The model under review builds one solid part; all positions refer to its coordinate system, in mm. A direction names the side the tool comes from. Round coordinates to 2 decimals unless told otherwise and drop trailing zeros. Order: outer loops, then holes, each group sorted by start corner. A loop starts at its lowest first (then second) coordinate and runs counter-clockwise, first axis right, second up. Notation, with made-up numbers: (-25, -13.75) -> (21, -13.75) arc R33 ccw to (21, 21.25) -> close; hole circle Ø1 at (51, 57). An arc over 180 degrees is marked (long way). Use a Markdown table: item, result. Add a question column.
```python
from build123d import *

# Parameters (mm, degrees)
PAD_DEPTH       = 28
SKETCH001_R     = 19
POCKET_DEPTH    = 5
POCKET001_DEPTH = 26
SKETCH003_W     = 30
SKETCH003_H     = 6
POCKET002_DEPTH = 10
SKETCH004_W     = 2.8
SKETCH004_H     = 40
PAD001_DEPTH    = 5.8
SKETCH005_W     = 2.722469
SKETCH005_H     = 3
SKETCH005_W_2   = 2.715425
PAD002_DEPTH    = 12
SKETCH006_R     = 1.6
POCKET003_DEPTH = 5
SKETCH007_W     = 1
SKETCH007_H     = 4
POCKET004_DEPTH = 6
PAD003_DEPTH    = 10
SKETCH009_W     = 14.845783
SKETCH009_H     = 0.4
POCKET005_DEPTH = 0.4


with BuildPart() as part:
    # Sketch → Pad (new body)
    with BuildSketch(Plane(origin=(0, 0, 0), x_dir=(1, 0, 0), z_dir=(0, 0, -1))):
        Polygon((-52.483848, 11.054775), (-10.483848, 11.054775), (-10.483848, 16.054775), (-24.483848, 32.054775), (-38.483848, 32.054775), (-52.483848, 16.054775), align=None)
    extrude(amount=PAD_DEPTH)

    # Sketch001 → Pocket (cut)
    with BuildSketch(Plane(origin=(0, -11.054775, 0), x_dir=(1, 0, 0), z_dir=(0, 1, 0))):
        with Locations((-31.483848, 21)):
            Circle(SKETCH001_R)
    extrude(amount=-POCKET_DEPTH, mode=Mode.SUBTRACT)

    # Sketch002 → Pocket001 (cut)
    with BuildSketch(Plane(origin=(0, 0, -28), x_dir=(1, 0, 0), z_dir=(0, 0, -1))):
        Polygon((-49.14737, 16.054775), (-36.483848, 32.054775), (-26.483848, 32.054775), (-13.820326, 16.054775), align=None)
    extrude(amount=-POCKET001_DEPTH, mode=Mode.SUBTRACT)

    # Sketch003 → Pocket002 (cut)
    with BuildSketch(Plane(origin=(0, 0, -28), x_dir=(1, 0, 0), z_dir=(0, 0, -1))):
        with Locations((-31.483848, 29.054775)):
            Rectangle(SKETCH003_W, SKETCH003_H)
    extrude(amount=-POCKET002_DEPTH, mode=Mode.SUBTRACT)

    # Sketch004 → Pad001 (new body)
    with BuildSketch(Plane(origin=(0, 0, -28), x_dir=(1, 0, 0), z_dir=(0, 0, -1))):
        with Locations((-46.98737, 40.454775)):
            Rectangle(SKETCH004_W, SKETCH004_H)
        with Locations((-15.98737, 40.454775)):
            Rectangle(SKETCH004_W, SKETCH004_H)
    extrude(amount=-PAD001_DEPTH)

    # Sketch005 → Pad002 (new body)
    with BuildSketch(Plane(origin=(0, 0, -28), x_dir=(1, 0, 0), z_dir=(0, 0, -1))):
        with Locations((-47.026135, 21.954775)):
            Rectangle(SKETCH005_W, SKETCH005_H)
        with Locations((-15.945082, 21.954775)):
            Rectangle(SKETCH005_W_2, SKETCH005_H)
    extrude(amount=-PAD002_DEPTH)

    # Sketch006 → Pocket003 (cut)
    with BuildSketch(Plane(origin=(0, -11.054775, 0), x_dir=(1, 0, 0), z_dir=(0, 1, 0))):
        with Locations((-47.483848, 4)):
            Circle(SKETCH006_R)
        with Locations((-15.483848, 4)):
            Circle(SKETCH006_R)
    extrude(amount=-POCKET003_DEPTH, mode=Mode.SUBTRACT)

    # Sketch007 → Pocket004 (cut)
    with BuildSketch(Plane(origin=(0, 0, -28), x_dir=(1, 0, 0), z_dir=(0, 0, -1))):
        with Locations((-46.98737, 55.054775)):
            Rectangle(SKETCH007_W, SKETCH007_H)
        with Locations((-15.98737, 55.054775)):
            Rectangle(SKETCH007_W, SKETCH007_H)
    extrude(amount=-POCKET004_DEPTH, mode=Mode.SUBTRACT)

    # Sketch008 → Pad003 (new body)
    with BuildSketch(Plane(origin=(0, 0, -18), x_dir=(1, 0, 0), z_dir=(0, 0, -1))):
        Polygon((-32.222141, 44.054382), (-31.422141, 44.054382), (-31.422141, 32.054775), (-24.483848, 32.054775), (-24.483848, 31.254775), (-38.483848, 31.254775), (-38.483848, 32.054775), (-32.222141, 32.054775), align=None)
    extrude(amount=PAD003_DEPTH)

    # Sketch009 → Pocket005 (cut)
    with BuildSketch(Plane(origin=(0, -31.254775, 0), x_dir=(1, 0, 0), z_dir=(0, 1, 0))):
        with Locations((-31.447088, 18.2)):
            Rectangle(SKETCH009_W, SKETCH009_H)
    extrude(amount=-POCKET005_DEPTH, mode=Mode.SUBTRACT)


solid = part.part
```
Q1. Add section A-A, the plane z = -21. Give the number of separate pieces and of enclosed holes in the cut face, then the cut area to 3 significant figures.
Q2. Add section D-D, the plane z = -4. Give the boundary of the cut face in (x, y), then the cut area to 3 significant figures.
Q3. For pin 1 (4.5 mm diameter, centred on y = -49.5, z = -24, fed in from +X); pin 2 (6 mm diameter, centred on x = -43.5, z = -7, fed in from -Y); pin 3 (2 mm diameter, centred on x = -21, z = -22.5, fed in from -Y), all flat-tipped, find the tip position at first contact; note any pin that passes through.
Q4. Draft analysis for pull direction X (two halves, no side actions). For faces 5 (the face through (-32.222, -38, -23)), 6 (the face through (-32, -35, -28)), 7 (the face through (-33, -32.055, -20)), 8 (the face through (-10.484, -14, -14)), state which applies: released by +X, released by -X, zero draft, split by the parting line, or undercut.
Q5. Add section C-C, the plane y = -33. Give the boundary of the cut face in (x, z), then the cut area to 3 significant figures.
Q6. To check wall thickness, follow line 1 along X through (y, z) = (-13.35, -21); line 2 along X through (y, z) = (-14.1, -4); line 3 along Z through (x, y) = (-34.5, -29). State the ranges of each line that lie inside material, in increasing order.
Q7. For faces 1 (the face through (-14.587, -22, -22)), 2 (the face through (-15.487, -55, -25)), 3 (the face through (-48.387, -22, -19)), 4 (the face through (-32.002, -13.52, -2.007)), list the 3-axis set-ups (+Z, -Z, +X, -X, +Y, -Y) from which the entire face can be reached by the end or side of a thin tool; tool diameter is ignored.
Q8. Add section B-B, the plane y = -55.5. Give the boundary of the cut face in (x, z), then the cut area to 3 significant figures.
Return value:
| question | item | result |
|---|---|---|
| 1 | separate pieces | 3 |
| 1 | enclosed holes | 0 |
| 1 | area | 106 mm² |
| 2 | outline | (-52.48, -16.05) -> (-38.48, -32.05) -> (-36.48, -32.05) -> (-49.15, -16.05) -> (-49.08, -16.05) -> (-49.08, -11.05) -> (-52.48, -11.05) -> close; (-45.88, -16.05) -> (-39.97, -16.05) -> (-39.97, -11.05) -> (-45.88, -11.05) -> close; (-26.48, -32.05) -> (-24.48, -32.05) -> (-10.48, -16.05) -> (-10.48, -11.05) -> (-13.88, -11.05) -> (-13.88, -16.05) -> (-13.82, -16.05) -> close; (-23, -16.05) -> (-17.08, -16.05) -> (-17.08, -11.05) -> (-23, -11.05) -> close |
| 2 | area | 179 mm² |
| 3 | pin 1 | x = -14.59 |
| 3 | pin 2 | y = -29.75 |
| 3 | pin 3 | y = -26.05 |
| 4 | face 5 | undercut |
| 4 | face 6 | zero draft |
| 4 | face 7 | undercut |
| 4 | face 8 | released by +X |
| 5 | outline | (-48.39, -28) -> (-45.59, -28) -> (-45.59, -22.2) -> (-48.39, -22.2) -> close; (-32.22, -28) -> (-31.42, -28) -> (-31.42, -18) -> (-32.22, -18) -> close; (-17.39, -28) -> (-14.59, -28) -> (-14.59, -22.2) -> (-17.39, -22.2) -> close |
| 5 | area | 40.5 mm² |
| 6 | line 1 | -52.48 to -50.48, -12.48 to -10.48 |
| 6 | line 2 | -52.48 to -49.08, -45.88 to -39.97, -23 to -17.08, -13.88 to -10.48 |
| 6 | line 3 | -2 to 0 |
| 7 | face 1 | +Z, -Z, +X, -Y |
| 7 | face 2 | +Z, -Z |
| 7 | face 3 | +Z, -Z, -X, -Y |
| 7 | face 4 | +Y |
| 8 | outline | (-48.39, -28) -> (-47.49, -28) -> (-47.49, -22.2) -> (-48.39, -22.2) -> close; (-46.49, -28) -> (-45.59, -28) -> (-45.59, -22.2) -> (-46.49, -22.2) -> close; (-17.39, -28) -> (-16.49, -28) -> (-16.49, -22.2) -> (-17.39, -22.2) -> close; (-15.49, -28) -> (-14.59, -28) -> (-14.59, -22.2) -> (-15.49, -22.2) -> close |
| 8 | area | 20.9 mm² |
